Input: part model. Units: mm. Frame: model coordinates. Face numbers are marked on the shaded views. A direction names the side the tool comes from. Round coordinates to 2 decimals unless told otherwise and drop trailing zeros. Order: outer loops, then holes, each group sorted by start corner. A loop starts at its lowest first (then second) coordinate and runs counter-clockwise, first axis right, second up. Notation, with made-up numbers: (-28.75, -14) -> (-11.75, -14) arc R26 ccw to (-11.75, 13) -> close; hole circle Ø9 at (31, 50). An arc over 180 degrees is marked (long way). Use a Markdown table: item, result.
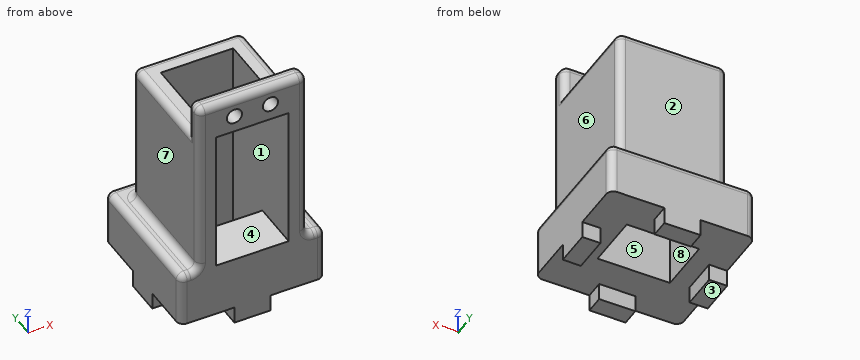
from build123d import *

# Parameters (mm, degrees)
SKETCH1_W           = 30
SKETCH1_H           = 33.5
SKETCH1_W_2         = 20
SKETCH1_H_2         = 23.5
BOSS_EXTRUDE1_DEPTH = 10
SKETCH1_4_W         = 30
SKETCH1_4_H         = 33.5
SKETCH1_4_W_2       = 20
SKETCH1_4_H_2       = 23.5
BOSS_EXTRUDE2_DEPTH = 5
SKETCH2_W           = 40
SKETCH2_H           = 38.5
BOSS_EXTRUDE3_DEPTH = 10
BOSS_EXTRUDE4_DEPTH = 40
SKETCH4_W           = 30
SKETCH4_H           = 5
BOSS_EXTRUDE5_DEPTH = 10
SKETCH5_R           = 2.1
CUT_EXTRUDE1_DEPTH  = 5
FILLET1_R           = 2
SKETCH6_W           = 10
SKETCH6_H           = 5
SKETCH6_W_2         = 5
SKETCH6_H_2         = 10
BOSS_EXTRUDE6_DEPTH = 4.7
SKETCH7_W           = 20
SKETCH7_H           = 15
CUT_EXTRUDE2_DEPTH  = 15


with BuildPart() as part:
    # Sketch1 → Boss-Extrude1 (new body)
    # profile 1 of 3: a face of its own
    with BuildSketch(Plane.XY):
        Polygon((-20, 19.25), (-20, -19.25), (-15, -19.25), (-15, 14.25), (15, 14.25), (15, -19.25), (20, -19.25), (20, 19.25), align=None)
    # profile 2 of 3: a face of its own
    with BuildSketch(Plane.XY):
        with Locations((0, -2.5)):
            Rectangle(SKETCH1_W, SKETCH1_H)
        with Locations((0, -2.5)):
            Rectangle(SKETCH1_W_2, SKETCH1_H_2, mode=Mode.SUBTRACT)
    # profile 3 of 3: a face of its own
    with BuildSketch(Plane.XY):
        with Locations((0, -2.5)):
            Rectangle(SKETCH1_W_2, SKETCH1_H_2)
    extrude(amount=-BOSS_EXTRUDE1_DEPTH)

    # Sketch1<4> → Boss-Extrude2 (add)
    with BuildSketch(Plane.XY):
        with Locations((0, -2.5)):
            Rectangle(SKETCH1_4_W, SKETCH1_4_H)
        with Locations((0, -2.5)):
            Rectangle(SKETCH1_4_W_2, SKETCH1_4_H_2, mode=Mode.SUBTRACT)
    extrude(amount=BOSS_EXTRUDE2_DEPTH)

    # Sketch2 → Boss-Extrude3 (add)
    with BuildSketch(Plane.XY.offset(5)):
        Rectangle(SKETCH2_W, SKETCH2_H)
    extrude(amount=-BOSS_EXTRUDE3_DEPTH)

    # Sketch3 → Boss-Extrude4 (add)
    with BuildSketch(Plane.XY.offset(5)):
        Polygon((-10, -19.25), (-10, -14.25), (-10, 9.25), (10, 9.25), (10, -14.25), (10, -19.25), (15, -19.25), (15, 14.25), (-15, 14.25), (-15, -19.25), align=None)
    extrude(amount=BOSS_EXTRUDE4_DEPTH)

    # Sketch4 → Boss-Extrude5 (add)
    with BuildSketch(Plane.XY.offset(45)):
        with Locations((0, -16.75)):
            Rectangle(SKETCH4_W, SKETCH4_H)
    extrude(amount=BOSS_EXTRUDE5_DEPTH)

    # Sketch5 → Cut-Extrude1 (cut)
    with BuildSketch(Plane.XZ.offset(19.25)):
        with Locations(Location((4.97, 49.66, 0), (0, 0, 270))):
            Circle(SKETCH5_R)
        with Locations(Location((-4.97, 49.66, 0), (0, 0, 270))):
            Circle(SKETCH5_R)
    extrude(amount=-CUT_EXTRUDE1_DEPTH, mode=Mode.SUBTRACT)

    # Fillet1
    fillet1_edges = [part.edges().sort_by_distance(p)[0] for p in [
        (-15, -14.25, 50),
        (15, -14.25, 50),
        (-15, -16.75, 55),
        (-20, 19.25, -2.5),
        (0, -19.25, 55),
        (15, -16.75, 55),
        (0, -14.25, 55),
        (20, 19.25, -2.5),
        (20, -19.25, -2.5),
        (-20, -19.25, -2.5),
        (-17.5, -19.25, 5),
        (20, 0, 5),
        (0, 19.25, 5),
        (-20, 0, 5),
        (17.5, -19.25, 5),
        (0, 14.25, 5),
        (15, 14.25, 25),
        (-15, -2.5, 5),
        (-15, 14.25, 25),
        (-15, -19.25, 30),
        (15, -2.5, 5),
        (15, -19.25, 30),
        (0, 14.25, 45),
        (-15, 0, 45),
        (15, 0, 45),
    ]]
    fillet(fillet1_edges, radius=FILLET1_R)

    # Sketch6 → Boss-Extrude6 (add)
    with BuildSketch(Plane(origin=(0, 0, -10), x_dir=(-1, 0, 0), z_dir=(0, 0, -1))):
        with Locations((0, -16.75)):
            Rectangle(SKETCH6_W, SKETCH6_H)
        with Locations((17.5, 0)):
            Rectangle(SKETCH6_W_2, SKETCH6_H_2)
        with Locations((0, 16.75)):
            Rectangle(SKETCH6_W, SKETCH6_H)
        with Locations((-17.5, 0)):
            Rectangle(SKETCH6_W_2, SKETCH6_H_2)
    extrude(amount=BOSS_EXTRUDE6_DEPTH)

    # Sketch7 → Cut-Extrude2 (cut)
    with BuildSketch(Plane.XY.offset(5)):
        with Locations((0, 1.75)):
            Rectangle(SKETCH7_W, SKETCH7_H)
    extrude(amount=-CUT_EXTRUDE2_DEPTH, mode=Mode.SUBTRACT)


solid = part.part
1) Cut plane B-B on z = 49.66. Return loops of the section in (x, y).
Answer key:
| item | result |
|---|---|
| outline | (-15, -17.25) arc R2 ccw to (-13, -19.25) -> (-7.07, -19.25) -> (-7.07, -14.25) -> (-13, -14.25) arc R2 ccw to (-15, -16.25) -> close; (-2.87, -19.25) -> (2.87, -19.25) -> (2.87, -14.25) -> (-2.87, -14.25) -> close; (7.07, -19.25) -> (13, -19.25) arc R2 ccw to (15, -17.25) -> (15, -16.25) arc R2 ccw to (13, -14.25) -> (7.07, -14.25) -> close |
2) Contact query for flat-ended pins moving along their axis: P1, Ø1.4, axis at y = 17.5, z = -12, coming from the -X side; P2, Ø1.4, axis at y = -16.5, z = -13.5, coming from the +X side; P3, Ø4, axis at x = 10, y = 13.5, coming from the +Z side. Output: stop coordinate, or through.
Answer key:
| item | result |
|---|---|
| P1 | stops at x = -5 |
| P2 | stops at x = 5 |
| P3 | stops at z = 45 |
3) Cut plane A-A on y = 0.5. Return loops of the section in (x, z).
Answer key:
| item | result |
|---|---|
| outline | (-20, -14.7) -> (-15, -14.7) -> (-15, -10) -> (-10, -10) -> (-10, 45) -> (-13, 45) arc R2 ccw to (-15, 43) -> (-15, 7) arc R2 cw to (-17, 5) -> (-18, 5) arc R2 ccw to (-20, 3) -> close; (10, -10) -> (15, -10) -> (15, -14.7) -> (20, -14.7) -> (20, 3) arc R2 ccw to (18, 5) -> (17, 5) arc R2 cw to (15, 7) -> (15, 43) arc R2 ccw to (13, 45) -> (10, 45) -> close |
4) Set-up query: the marked faces 5, 6, 7 and 8. Return all of +Z, -Z, +X, -X, +Y, -Y with unobstructed straight access to the full face (end or side cutting, diameter ignored); none if empty.
Answer key:
| item | result |
|---|---|
| face 5 | +Z, -Z |
| face 6 | +Z, +X, +Y, -Y |
| face 7 | +Z, -X, +Y, -Y |
| face 8 | none |
5) Draft query along Z for the marked faces 1, 2, 3 and 4. Return one class per face: released by +Z, released by -Z, zero draft, split by the parting line, or undercut.
Answer key:
| item | result |
|---|---|
| face 1 | undercut |
| face 2 | zero draft |
| face 3 | released by -Z |
| face 4 | undercut |
6) Cut plane C-C on z = 17.5. Return loops of the section in (x, y).
Answer key:
| item | result |
|---|---|
| outline | (-15, -17.25) arc R2 ccw to (-13, -19.25) -> (-10, -19.25) -> (-10, 9.25) -> (10, 9.25) -> (10, -19.25) -> (13, -19.25) arc R2 ccw to (15, -17.25) -> (15, 12.25) arc R2 ccw to (13, 14.25) -> (-13, 14.25) arc R2 ccw to (-15, 12.25) -> close |
7) Ray query, probe 1 along X at (y, z) = (-17, 43.5); probe 2 along X at (y, z) = (-16.3, 49.66); probe 3 along X at (y, z) = (-15.6, 49.66). Return the intervals inside material, ascending.
Answer key:
| item | result |
|---|---|
| probe 1 | x = -15 to -10, 10 to 15 |
| probe 2 | x = -15 to -7.07, -2.87 to 2.87, 7.07 to 15 |
| probe 3 | x = -14.89 to -7.07, -2.87 to 2.87, 7.07 to 14.89 |
8) Cut plane D-D on y = 7. Return loops of the section in (x, z), and give its area (3 significant figures).
Answer key:
| item | result |
|---|---|
| outline | (-20, -10) -> (-10, -10) -> (-10, 45) -> (-13, 45) arc R2 ccw to (-15, 43) -> (-15, 7) arc R2 cw to (-17, 5) -> (-18, 5) arc R2 ccw to (-20, 3) -> close; (10, -10) -> (20, -10) -> (20, 3) arc R2 ccw to (18, 5) -> (17, 5) arc R2 cw to (15, 7) -> (15, 43) arc R2 ccw to (13, 45) -> (10, 45) -> close |
| area | 698 mm^2 |
